Source: CAD feature listing. Evaluate the final solid. Frame: model axes, mm. Face numbers are marked on the shaded views. A direction names the side the tool comes from. Give positions to 0.01 mm unless a question says otherwise; leave off trailing zeros. Write each loop counter-clockwise with the first axis right and the second up, starting at its lowest first coordinate (ties: lowest second). Pieces come first, ordered by that corner, then holes.
```python
from build123d import *

# Parameters (mm, degrees)
BOSS_EXTRUDE1_DEPTH = 380
SKETCH2_W           = 4
SKETCH2_H           = 9
CUT_EXTRUDE1_DEPTH  = 1.5
BOSS_EXTRUDE2_DEPTH = 380


with BuildPart() as part:
    # Sketch1 → Boss-Extrude1 (new body)
    with BuildSketch(Plane(origin=(0, 0, 0), x_dir=(1, 0, 0), z_dir=(0, 1, 0))):
        with BuildLine():
            Line((0, 48.5), (-97.832794656, 48.5))
            ThreePointArc((-97.832794656, 48.5), (-107.732532415, 44.769214361), (-112.707763578, 35.432692308))
            ThreePointArc((-112.707763578, 35.432692308), (-115, 0), (-112.707763578, -35.432692308))
            ThreePointArc((-112.707763578, -35.432692308), (-107.732532415, -44.769214361), (-97.832794656, -48.5))
            Line((-97.832794656, -48.5), (0, -48.5))
            Line((0, -48.5), (0, -45.5))
            Line((0, -45.5), (-97.832794656, -45.5))
            ThreePointArc((-97.832794656, -45.5), (-105.752584863, -42.515371489), (-109.732769794, -35.046153846))
            ThreePointArc((-109.732769794, -35.046153846), (-112, 0), (-109.732769794, 35.046153846))
            ThreePointArc((-109.732769794, 35.046153846), (-105.752584863, 42.515371489), (-97.832794656, 45.5))
            Line((-97.832794656, 45.5), (0, 45.5))
            Line((0, 45.5), (0, 48.5))
        make_face()
    extrude(amount=BOSS_EXTRUDE1_DEPTH)

    # Sketch2 → Cut-Extrude1 (cut)
    with BuildSketch(Plane.XY.offset(-45.5)):
        with Locations((-92.832794656, 380)):
            Rectangle(SKETCH2_W, SKETCH2_H)
        with Locations((-25.832794656, 380)):
            Rectangle(SKETCH2_W, SKETCH2_H)
    cut_extrude1 = extrude(amount=-CUT_EXTRUDE1_DEPTH, mode=Mode.SUBTRACT)

    # Mirror1: Cut-Extrude1 across plane
    add(cut_extrude1.mirror(Plane.XY), mode=Mode.SUBTRACT)

    # Sketch3 → Boss-Extrude2 (add)
    with BuildSketch(Plane(origin=(0, 0, 0), x_dir=(1, 0, 0), z_dir=(0, 1, 0))):
        with BuildLine():
            Line((0, 0), (0, 31.952645856))
            ThreePointArc((0, 31.952645856), (-0.585786438, 33.366859418), (-2, 33.952645856))
            Line((-2, 33.952645856), (-10.490338609, 33.952645856))
            Line((-10.490338609, 33.952645856), (-15.497576902, 38.606995774))
            Line((-15.497576902, 38.606995774), (-15.497576902, 45.5))
            Line((-15.497576902, 45.5), (-16.497576902, 45.5))
            Line((-16.497576902, 45.5), (-16.497576902, 38.171230588))
            Line((-16.497576902, 38.171230588), (-10.88332405, 32.952645856))
            Line((-10.88332405, 32.952645856), (-2, 32.952645856))
            ThreePointArc((-2, 32.952645856), (-1.292893219, 32.659752637), (-1, 31.952645856))
            Line((-1, 31.952645856), (-1, 0))
            Line((-1, 0), (-1, -31.952645856))
            ThreePointArc((-1, -31.952645856), (-1.292893219, -32.659752637), (-2, -32.952645856))
            Line((-2, -32.952645856), (-10.88332405, -32.952645856))
            Line((-10.88332405, -32.952645856), (-16.497576902, -38.171230588))
            Line((-16.497576902, -38.171230588), (-16.497576902, -45.5))
            Line((-16.497576902, -45.5), (-15.497576902, -45.5))
            Line((-15.497576902, -45.5), (-15.497576902, -38.606995774))
            Line((-15.497576902, -38.606995774), (-10.490338609, -33.952645856))
            Line((-10.490338609, -33.952645856), (-2, -33.952645856))
            ThreePointArc((-2, -33.952645856), (-0.585786438, -33.366859418), (0, -31.952645856))
            Line((0, -31.952645856), (0, 0))
        make_face()
    extrude(amount=BOSS_EXTRUDE2_DEPTH)


solid = part.part
```
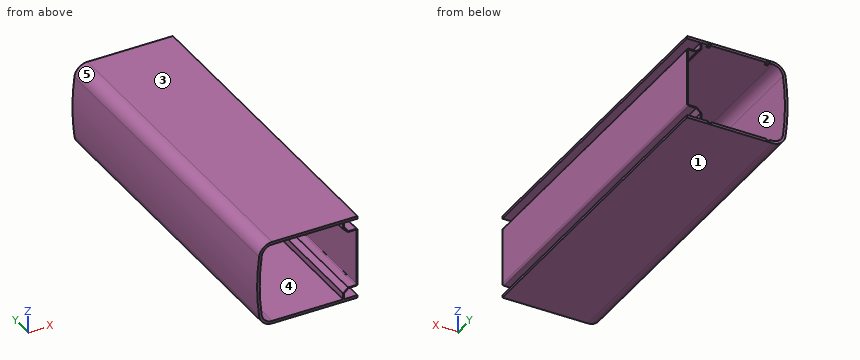
1. Line query: L1, parallel to Z at x = -7.5, y = 27; L2, parallel to Z at x = -84, y = 140; L3, parallel to X at y = 351, z = -3. Output: solid intervals per line, ascending.
2. Access query for the marked faces 1 and 2. Directions: +Z, -Z, +X, -X, +Y, -Y. A direction counts if a zero-diameter tool reaches every point of the face in a straight line with its end or side. Return the directions, or none.
3. Cut plane B-B, the plane x = -75. Return the cut outline in (y, z).
4. Cut plane C-C, the plane z = 1. Return the cut outline in (x, y).
5. Mould query, pull axis X, two halves, no side actions, for the marked faces 3, 4 and 5. Classes: +X half, -X half, draft (parallel to the pull), parting line (faces both ways), or undercut.
6. Contact query for flat-ended pins moving along their axis: P1, Ø1.2, axis at y = 377.5, z = 46, coming from the -X side; P2, Ø6, axis at y = 241.5, z = -42.5, coming from the -X side; P3, Ø0.8, axis at y = 378, z = 46.5, coming from the -X side. Output: stop coordinate, or through.
Response values:
1. L1: z = -48.5 to -45.5, -33.95 to -32.95, 32.95 to 33.95, 45.5 to 48.5
1. L2: z = -48.5 to -45.5, 45.5 to 48.5
1. L3: x = -114.98 to -111.98, -1 to 0
2. face 1: -Z, +X, -X, +Y, -Y
2. face 2: +Y, -Y
3. outline: (0, -48.5) - (380, -48.5) - (380, -45.5) - (0, -45.5) - close; (0, 45.5) - (380, 45.5) - (380, 48.5) - (0, 48.5) - close
4. outline: (-115, 0) - (-112, 0) - (-112, 380) - (-115, 380) - close; (-1, 0) - (0, 0) - (0, 380) - (-1, 380) - close
5. face 3: draft
5. face 4: undercut
5. face 5: -X half
6. P1: stops at x = -106.96
6. P2: stops at x = -111.58
6. P3: stops at x = -105.97
